Build history of the part. All positions in model axes, mm. Face numbers are marked on the shaded views. A direction names the side the tool comes from. Round coordinates to 2 decimals unless told otherwise and drop trailing zeros. Loops run counter-clockwise (first coordinate to the right, second up) from the corner with the lowest first, then second, coordinate; pieces in that order, holes last.
from build123d import *

# Parameters (mm, degrees)
F0_W      = 12.420304
F0_H      = 81.656884
F1_DEPTH  = 2.5
F2_DEPTH  = 1.5
F1_FACE_W = 12.420304
F1_FACE_H = 81.656884
F3_DEPTH  = 5
F4_DEPTH  = 2


with BuildPart() as f1:
    # F0 (on Top) → F1 (new body)
    with BuildSketch(Plane.XY):
        with Locations((-46.245806, 10.306211)):
            Rectangle(F0_W, F0_H)
    extrude(amount=F1_DEPTH)

    # F0 (on Top) → F2 (join)
    with BuildSketch(Plane.XY):
        Polygon((-46.113677, 61.70512), (-52.455958, 51.134653), (-40.035654, 51.134653), align=None)
    extrude(amount=F2_DEPTH)

    # F1_face (on face) → F3 (join)
    with BuildSketch(Plane(origin=(-46.245806, 10.306211, 2.5), x_dir=(1, 0, 0), z_dir=(0, 0, 1))):
        Rectangle(F1_FACE_W, F1_FACE_H)
    extrude(amount=-F3_DEPTH)

    # F0 (on Top) → F4 (join)
    with BuildSketch(Plane.XY):
        Polygon((-46.113677, 61.70512), (-52.455958, 51.134653), (-40.035654, 51.134653), align=None)
    extrude(amount=-F4_DEPTH)


solid = f1.part
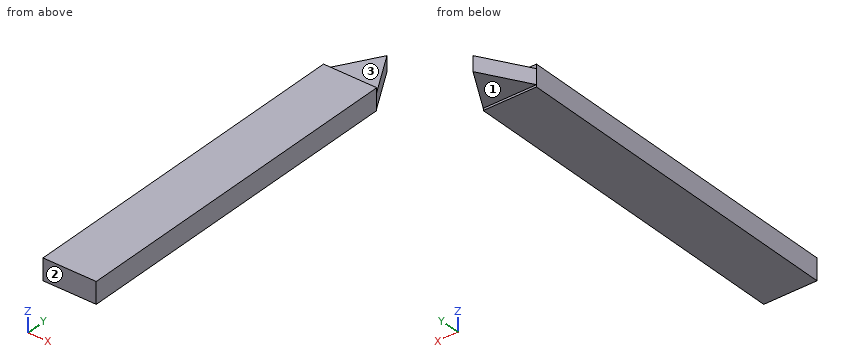
(1) Slice it at B-B on z = 0.4. List the corners of the cut face in (x, y), plus the area to 3 significant figures.
Responses:
outline: (-52.46, -30.52) - (-40.04, -30.52) - (-40.04, 51.13) - (-46.11, 61.71) - (-52.46, 51.13) - close
area: 1,080 mm2
(2) Pin check, flat tips, straight feed: P1, Ø5.5, axis at x = -49, y = 57, coming from the +Z side; P2, Ø1, axis at x = -45, z = -2, coming from the +Y side; P3, Ø2, axis at x = -41.5, z = -0.5, coming from the +Y side. Stop position of each tip, or through.
Responses:
P1: stops at z = 1.5
P2: stops at y = 60.64
P3: stops at y = 55.42
(3) Slice it at A-A on x = -41.75. List the corners of the cut face in (y, z).
Responses:
outline: (-30.52, -2.5) - (51.13, -2.5) - (51.13, -2) - (54.12, -2) - (54.12, 1.5) - (51.13, 1.5) - (51.13, 2.5) - (-30.52, 2.5) - close
(4) Which spindle directions (+Z, -Z, +X, -X, +Y, -Y) get a long thin tool onto all of the face, cutting with end or side? Do the marked faces 1, 2 and 3. Say none if no direction does.
Responses:
face 1: -Z, +X, -X, +Y
face 2: +Z, -Z, +X, -X, -Y
face 3: +Z, +X, -X, +Y
(5) Probe line 1 (Z direction, x = -44.75, y = 52); line 2 (Y direction, x = -49, z = 1.65); line 3 (Y direction, x = -44.5, z = 1.1). List the from-to ranges inside material, lowest first.
Responses:
line 1: z = -2 to 1.5
line 2: y = -30.52 to 51.13
line 3: y = -30.52 to 58.9
(6) Slice it at C-C on x = -50.75. List the corners of the cut face in (y, z), plus the area to 3 significant figures.
Responses:
outline: (-30.52, -2.5) - (51.13, -2.5) - (51.13, -2) - (53.98, -2) - (53.98, 1.5) - (51.13, 1.5) - (51.13, 2.5) - (-30.52, 2.5) - close
area: 418 mm2
